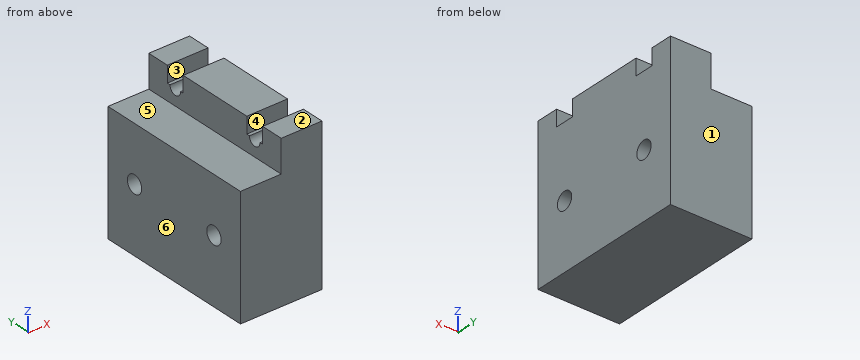
from build123d import *

# Parameters (mm, degrees)
F0_W             = 25
F0_H             = 47
F1_DEPTH         = 25
F4_D             = 5.4102
F4_DEPTH         = 10
F4_TIP           = 1.6253880605
F4_ON_F3_D       = 5.4102
F4_ON_F3_DEPTH   = 10
F4_ON_F3_TIP     = 1.6253880605
F5_W             = 12.5
F5_H             = 10
F6_DEPTH         = 50.001
F7_W             = 12.5
F7_H             = 6
F8_DEPTH         = 5
F11_D            = 2.4
F11_DEPTH        = 10
F11_TIP          = 0.7210327428
F11_ON_F10_D     = 2.4
F11_ON_F10_DEPTH = 10
F11_ON_F10_TIP   = 0.7210327428
F9_W             = 7
F9_H             = 2
F10_W            = 7
F10_H            = 2


with BuildPart() as f1:
    # F0 (on Front) → F1 (new body, symmetric)
    with BuildSketch(Plane.XZ):
        with Locations((0, 3.5)):
            Rectangle(F0_W, F0_H)
    extrude(amount=F1_DEPTH, both=True)

    # F4
    with Locations(Plane(origin=(-12.5, 0, 0), x_dir=(0, -1, 0), z_dir=(-1, 0, 0))):
        with Locations((-15, 0), (15, 0)):
            Hole(F4_D / 2, depth=F4_DEPTH)
            with Locations((0, 0, -(F4_DEPTH + F4_TIP / 2))):  # 118° drill point
                Cone(0, F4_D / 2, F4_TIP, mode=Mode.SUBTRACT)

    # F4 on F3
    with Locations(Plane.YZ.offset(12.5)):
        with Locations((-15, 0), (15, 0)):
            Hole(F4_ON_F3_D / 2, depth=F4_ON_F3_DEPTH)
            with Locations((0, 0, -(F4_ON_F3_DEPTH + F4_ON_F3_TIP / 2))):  # 118° drill point
                Cone(0, F4_ON_F3_D / 2, F4_ON_F3_TIP, mode=Mode.SUBTRACT)

    # F5 (on face) → F6 (cut, through all)
    with BuildSketch(Plane.XZ.offset(25)):
        with Locations((-6.25, 22)):
            Rectangle(F5_W, F5_H)
    extrude(amount=-F6_DEPTH, mode=Mode.SUBTRACT)

    # F7 (on face) → F8 (cut)
    with BuildSketch(Plane.XY.offset(27)):
        with Locations((6.25, 15)):
            Rectangle(F7_W, F7_H)
        with Locations((6.25, -15)):
            Rectangle(F7_W, F7_H)
    extrude(amount=-F8_DEPTH, mode=Mode.SUBTRACT)

    # F11
    with Locations(Plane.XY.offset(22)):
        with Locations((9, 15)):
            Hole(F11_D / 2, depth=F11_DEPTH)
            with Locations((0, 0, -(F11_DEPTH + F11_TIP / 2))):  # 118° drill point
                Cone(0, F11_D / 2, F11_TIP, mode=Mode.SUBTRACT)

    # F11 on F10
    with Locations(Plane.XY.offset(22)):
        with Locations((9, -15)):
            Hole(F11_ON_F10_D / 2, depth=F11_ON_F10_DEPTH)
            with Locations((0, 0, -(F11_ON_F10_DEPTH + F11_ON_F10_TIP / 2))):  # 118° drill point
                Cone(0, F11_ON_F10_D / 2, F11_ON_F10_TIP, mode=Mode.SUBTRACT)

    # F9 (on face) → F12 (revolve, cut)
    with BuildSketch(Plane.XY.offset(22)):
        with Locations((3.5, 16)):
            Rectangle(F9_W, F9_H)
    revolve(axis=Axis((7.6713971794, 15, 22), (1, 0, 0)), mode=Mode.SUBTRACT)

    # F10 (on face) → F13 (revolve, cut)
    with BuildSketch(Plane.XY.offset(22)):
        with Locations((3.5, -14)):
            Rectangle(F10_W, F10_H)
    revolve(axis=Axis((7.2402027436, -15, 22), (1, 0, 0)), mode=Mode.SUBTRACT)


solid = f1.part
Source: CAD feature listing. Evaluate the final solid. Frame: model axes, mm. Face numbers are marked on the shaded views. A direction names the side the tool comes from. Round coordinates to 2 decimals unless told otherwise and drop trailing zeros. Loops run counter-clockwise (first coordinate to the right, second up) from the corner with the lowest first, then second, coordinate; pieces in that order, holes last. Notation, with made-up numbers: (62.5, 70.5) -> (108.5, 70.5) arc R12 ccw to (108.5, 79.5) -> close; hole circle Ø3 at (10, 17). An arc over 180 degrees is marked (long way). Answer as a JSON object with one key per item and string values. Group by question number.
Q1. Section query B-B (z = 18). Output: boundary loops of the cut face in (x, y).
Q2. Ray query, line 1 (Y direction, x = 7.25, z = 0); line 2 (Y direction, x = 9, z = 14.5); line 3 (X direction, y = 15, z = 18.25). Return the intervals inside material, ascending. Write a range as from..to.
Q3. Section query C-C (y = 20). Output: boundary loops of the cut face in (x, z).
Q4. Section query D-D (x = -6). Output: boundary loops of the cut face in (y, z), plus the area to 3 significant figures.
Q5. Access query for the marked faces 5 and 6. Directions: +Z, -Z, +X, -X, +Y, -Y. A direction counts if a zero-diameter tool reaches every point of the face in a straight line with its end or side. Return the directions, or none.
Q6. Section query A-A (x = 5.75). Output: boundary loops of the cut face in (y, z), plus the area to 3 significant figures.
Q7. Mould query, pull axis Y, two halves, no side actions, for the marked faces 1, 2, 3 and 4. Classes: pulls with the +Y half, pulls with the -Y half, needs draft (parallel to the pull), parting line crosses it, or undercut.
Q8. Contact query for flat-ended pins moving along their axis: P1, Ø5, axis at y = 15, z = 0, coming from the -X side; P2, Ø6, axis at x = -6, y = 5.5, coming from the +Z side; P3, Ø8, axis at y = 9.5, z = 21.5, coming from the -X side. Output: stop coordinate, or through.
Completed:
{
 "1": {"outline": "(0, -25) -> (12.5, -25) -> (12.5, 25) -> (0, 25) -> close; hole circle Ø2.4 at (9, -15); hole circle Ø2.4 at (9, 15)"},
 "2": {"line 1": "-25..-17.71, -12.29..12.29, 17.71..25", "line 2": "-25..-16.2, -13.8..13.8, 16.2..25", "line 3": "0..7.8, 10.2..12.5"},
 "3": {"outline": "(-12.5, -20) -> (12.5, -20) -> (12.5, 27) -> (0, 27) -> (0, 17) -> (-12.5, 17) -> close"},
 "4": {"outline": "(-25, -20) -> (25, -20) -> (25, 17) -> (-25, 17) -> close; hole circle Ø5.41 at (-15, 0); hole circle Ø5.41 at (15, 0)", "area": "1,800 mm²"},
 "5": {"face 5": "+Z, -X, +Y, -Y", "face 6": "+Z, -Z, -X, +Y, -Y"},
 "6": {"outline": "(-25, -20) -> (25, -20) -> (25, 27) -> (18, 27) -> (18, 22) -> (17, 22) arc R2 cw to (13, 22) -> (12, 22) -> (12, 27) -> (-12, 27) -> (-12, 22) -> (-13, 22) arc R2 cw to (-17, 22) -> (-18, 22) -> (-18, 27) -> (-25, 27) -> close; hole circle Ø5.41 at (-15, 0); hole circle Ø5.41 at (15, 0)", "area": "2,230 mm²"},
 "7": {"face 1": "pulls with the +Y half", "face 2": "needs draft", "face 3": "undercut", "face 4": "undercut"},
 "8": {"P1": "x = -2.38", "P2": "z = 17", "P3": "x = 0"}
}
